```python
from build123d import *

# Parameters (mm, degrees)
SKETCH1_W           = 28.575
SKETCH1_H           = 31.75
BOSS_EXTRUDE1_DEPTH = 3.5
SKETCH3_R           = 2
CUT_EXTRUDE1_DEPTH  = 6


with BuildPart() as part:
    # Sketch1 → Boss-Extrude1 (new, symmetric)
    with BuildSketch(Plane.XY):
        Rectangle(SKETCH1_W, SKETCH1_H)
    extrude(amount=BOSS_EXTRUDE1_DEPTH, both=True)

    # Sketch3 → Cut-Extrude1 (cut)
    with BuildSketch(Plane(origin=(0, 15.875, 0), x_dir=(1, 0, 0), z_dir=(0, 1, 0))):
        with Locations(Location((-10, 0, 0), (0, 0, 270))):
            Circle(SKETCH3_R)
        with Locations(Location((10, 0, 0), (0, 0, 90))):
            Circle(SKETCH3_R)
    extrude(amount=-CUT_EXTRUDE1_DEPTH, mode=Mode.SUBTRACT)


solid = part.part
```
Geometry check sheet. Reference: the model listing, model coordinates, mm. A direction names the side the tool comes from. Coordinates: 2 decimals unless noted, no trailing zeros. Order: outer loops, then holes, each group sorted by start corner. A loop starts at its lowest first (then second) coordinate and runs counter-clockwise, first axis right, second up. Notation, with made-up numbers: (66, 41) - (72, 41) arc R14 ccw to (72, 63) - close; hole circle Ø8 at (45.5, 20). An arc over 180 degrees is marked (long way). Answer in a Markdown table with one row per item. Add a question column.
1. Material ranges on L1, parallel to X at y = 12.9, z = 0; L2, parallel to Y at x = 11.5, z = 1.25 (3 decimals); L3, parallel to Z at x = 10, y = 12.2, recorded low to high. Write a range as [from, to].
2. Section check B-B (z = 0). Enter the section's corners in (x, y) (1 decimal), plus the area to 3 significant figures.
3. Draft check along Z on faces 1 (the face through (0, 0, -3.5)), 2 (the face through (0, 0, 3.5)), 3 (the face through (-8, 13, 0)), 4 (the face through (0, 15.875, 0)). Enter one of: +Z half, -Z half, draft (parallel to the pull), parting line (faces both ways), or undercut.
4. Access from +Z, -Z, +X, -X, +Y, -Y to the whole of each face (thin tool, end or side, straight path). Record for faces 5 (the face through (8, 13, 0)), 6 (the face through (0, -15.875, 0)).
5. Gauge pin test, flat end, axial feed: pin 1 Ø1.2 at (x, z) = (9.5, 1) entering from +Y (3 decimals). Record the tip position at first contact, or that the pin passes through.
6. Section check A-A (x = 10). Enter the section's corners in (y, z) (3 decimals), plus the area to 3 significant figures.
Data:
| question | item | result |
|---|---|---|
| 1 | L1 | x = [-14.29, -12], [-8, 8], [12, 14.29] |
| 1 | L2 | y = [-15.875, 9.875] |
| 1 | L3 | z = [-3.5, -2], [2, 3.5] |
| 2 | outline | (-14.3, -15.9) - (14.3, -15.9) - (14.3, 15.9) - (12, 15.9) - (12, 9.9) - (8, 9.9) - (8, 15.9) - (-8, 15.9) - (-8, 9.9) - (-12, 9.9) - (-12, 15.9) - (-14.3, 15.9) - close |
| 2 | area | 859 mm² |
| 3 | face 1 | -Z half |
| 3 | face 2 | +Z half |
| 3 | face 3 | undercut |
| 3 | face 4 | draft |
| 4 | face 5 | +Y |
| 4 | face 6 | +Z, -Z, +X, -X, -Y |
| 5 | pin 1 | stops at y = 9.875 |
| 6 | outline | (-15.875, -3.5) - (15.875, -3.5) - (15.875, -2) - (9.875, -2) - (9.875, 2) - (15.875, 2) - (15.875, 3.5) - (-15.875, 3.5) - close |
| 6 | area | 198 mm² |
